from build123d import *

# Parameters (mm, degrees)
BOSS_EXTRUDE1_DEPTH                                 = 6.35
BOSS_EXTRUDE1_DEPTH_BACK                            = 0.762
BOSS_EXTRUDE2_DEPTH                                 = 42.418
CSK_FOR_1_4_FLAT_HEAD_MACHINE_SCREW_100_D           = 6.7564
CSK_FOR_1_4_FLAT_HEAD_MACHINE_SCREW_100_CSINK_D     = 14.3913352
CSK_FOR_1_4_FLAT_HEAD_MACHINE_SCREW_100_CSINK_ANGLE = 100
FILLET1_R                                           = 1.27
CHAMFER1_SIZE                                       = 1.27
FILLET2_R                                           = 1.27


with BuildPart() as part:
    # Sketch2 → Boss-Extrude1 (new, two sides: drawn at the far end of the back side and taken through both)
    with BuildSketch(Plane(origin=(0, 43.18, 0), x_dir=(1, 0, 0), z_dir=(0, 1, 0)).offset(-BOSS_EXTRUDE1_DEPTH_BACK)):
        with BuildLine():
            Line((-27.94, 15.875), (-27.94, -15.875))
            ThreePointArc((-27.94, -15.875), (-24.406243315, -24.406243315), (-15.875, -27.94))
            Line((-15.875, -27.94), (15.875, -27.94))
            ThreePointArc((15.875, -27.94), (24.406243315, -24.406243315), (27.94, -15.875))
            Line((27.94, -15.875), (27.94, 15.875))
            ThreePointArc((27.94, 15.875), (24.406243315, 24.406243315), (15.875, 27.94))
            Line((15.875, 27.94), (-15.875, 27.94))
            ThreePointArc((-15.875, 27.94), (-24.406243315, 24.406243315), (-27.94, 15.875))
        make_face()
    extrude(amount=BOSS_EXTRUDE1_DEPTH + BOSS_EXTRUDE1_DEPTH_BACK)

    # Sketch1 → Boss-Extrude2 (add)
    with BuildSketch(Plane(origin=(0, 0, 0), x_dir=(1, 0, 0), z_dir=(0, 1, 0))):
        with BuildLine():
            Line((-27.94, -15.875), (-27.94, 15.875))
            ThreePointArc((-27.94, 15.875), (-24.406243315, 24.406243315), (-15.875, 27.94))
            Line((-15.875, 27.94), (15.875, 27.94))
            ThreePointArc((15.875, 27.94), (24.406243315, 24.406243315), (27.94, 15.875))
            Line((27.94, 15.875), (27.94, -15.875))
            ThreePointArc((27.94, -15.875), (24.406243315, -24.406243315), (15.875, -27.94))
            Line((15.875, -27.94), (-15.875, -27.94))
            ThreePointArc((-15.875, -27.94), (-24.406243315, -24.406243315), (-27.94, -15.875))
        make_face()
        with BuildLine():
            Line((-22.86, -15.875), (-22.86, 15.875))
            ThreePointArc((-22.86, 15.875), (-20.814140867, 20.814140867), (-15.875, 22.86))
            Line((-15.875, 22.86), (15.875, 22.86))
            ThreePointArc((15.875, 22.86), (20.814140867, 20.814140867), (22.86, 15.875))
            Line((22.86, 15.875), (22.86, -15.875))
            ThreePointArc((22.86, -15.875), (20.814140867, -20.814140867), (15.875, -22.86))
            Line((15.875, -22.86), (-15.875, -22.86))
            ThreePointArc((-15.875, -22.86), (-20.814140867, -20.814140867), (-22.86, -15.875))
        make_face(mode=Mode.SUBTRACT)
    extrude(amount=BOSS_EXTRUDE2_DEPTH)

    # CSK for 1/4 Flat Head Machine Screw (100)1 (through all)
    with Locations(Plane(origin=(0, 49.53, 0), x_dir=(1, 0, 0), z_dir=(0, 1, 0))):
        with Locations((0, 0)):
            CounterSinkHole(CSK_FOR_1_4_FLAT_HEAD_MACHINE_SCREW_100_D / 2, CSK_FOR_1_4_FLAT_HEAD_MACHINE_SCREW_100_CSINK_D / 2, counter_sink_angle=CSK_FOR_1_4_FLAT_HEAD_MACHINE_SCREW_100_CSINK_ANGLE)

    # Fillet1
    fillet1_edges = [part.edges().sort_by_distance(p)[0] for p in [
        (24.406243315, 49.53, 24.406243315),
        (27.94, 49.53, 0),
        (24.406243315, 49.53, -24.406243315),
        (0, 49.53, -27.94),
        (-24.406243315, 49.53, -24.406243315),
        (-27.94, 49.53, 0),
        (-24.406243315, 49.53, 24.406243315),
        (0, 49.53, 27.94),
    ]]
    fillet(fillet1_edges, radius=FILLET1_R)

    # Chamfer1
    chamfer1_edges = [part.edges().sort_by_distance(p)[0] for p in [
        (-22.86, 0, 0),
        (-20.814140867, 0, 20.814140867),
        (0, 0, 22.86),
        (20.814140867, 0, 20.814140867),
        (22.86, 0, 0),
        (20.814140867, 0, -20.814140867),
        (0, 0, -22.86),
        (-20.814140867, 0, -20.814140867),
    ]]
    chamfer(chamfer1_edges, length=CHAMFER1_SIZE)

    # Fillet2
    fillet2_edges = [part.edges().sort_by_distance(p)[0] for p in [
        (-27.94, 0, 0),
        (-24.406243315, 0, -24.406243315),
        (0, 0, -27.94),
        (24.406243315, 0, -24.406243315),
        (27.94, 0, 0),
        (24.406243315, 0, 24.406243315),
        (0, 0, 27.94),
        (-24.406243315, 0, 24.406243315),
    ]]
    fillet(fillet2_edges, radius=FILLET2_R)


solid = part.part
Check sheet for the modelled part. Datum: model origin and axes. Units: mm. A direction names the side the tool comes from. Round coordinates to 2 decimals unless told otherwise and drop trailing zeros. Write each loop counter-clockwise with the first axis right and the second up, starting at its lowest first coordinate (ties: lowest second). Pieces come first, ordered by that corner, then holes. Notation, with made-up numbers: (75, -11.5) -> (121, -11.5) arc R22 cw to (121, 18.5) -> close; hole circle Ø3 at (-33.5, 39). An arc over 180 degrees is marked (long way). Answer as CSV lines item,"result". Start each with the question number.
1) Go/stop test with flat-tipped pins: P1, Ø6, axis at x = 3, z = -2, coming from the +Y side; P2, Ø1, axis at x = 2.5, z = 14, coming from the -Y side. Record where each tip stops, or that it passes through.
2) Section check A-A on x = 0. Enter the section's corners in (y, z), and give its area (3 significant figures).
3) Section check D-D on x = 8. Enter the section's corners in (y, z), and give its area (3 significant figures).
4) Tool access check on faces 1 (the conical face through (-21.01, 1.07, -20.9)), 2 (the conical face through (-3.3, 46.5, 1.4)). Record the directions out of +Z, -Z, +X, -X, +Y, -Y that give a thin tool (end or side, any length) a straight path to the whole face; none if there is none.
5) Section check C-C on y = 23.5. Enter the section's corners in (x, z) (3 decimals).
6) Material ranges on line 1 (Z direction, x = 10, y = 18.5); line 2 (Z direction, x = 0, y = 43), recorded low to high. Write a range as from..to.
7) Section check B-B on z = 0. Enter the section's corners in (x, y).
8) Release check for a two-part mould opening along X. For faces 3 (the flat face through (26, 0, 0)), 4 (the cylindrical face through (24.31, 24.44, -24.5)), 5 (the flat face through (0, 22, -22.86)) record: pulls with the +X half, pulls with the -X half, needs draft (parallel to the pull), parting line crosses it, or undercut.
Found:
1,P1,"stops at y = 49.03"
1,P2,"stops at y = 42.42"
2,outline,"(0, -26.67) arc R1.27 ccw to (1.27, -27.94) -> (48.26, -27.94) arc R1.27 ccw to (49.53, -26.67) -> (49.53, -7.2) -> (46.33, -3.38) -> (42.42, -3.38) -> (42.42, -22.86) -> (1.27, -22.86) -> (0, -24.13) -> close; (0, 24.13) -> (1.27, 22.86) -> (42.42, 22.86) -> (42.42, 3.38) -> (46.33, 3.38) -> (49.53, 7.2) -> (49.53, 26.67) arc R1.27 ccw to (48.26, 27.94) -> (1.27, 27.94) arc R1.27 ccw to (0, 26.67) -> close"
2,area,"765 mm^2"
3,outline,"(0, -26.67) arc R1.27 ccw to (1.27, -27.94) -> (48.26, -27.94) arc R1.27 ccw to (49.53, -26.67) -> (49.53, 26.67) arc R1.27 ccw to (48.26, 27.94) -> (1.27, 27.94) arc R1.27 ccw to (0, 26.67) -> (0, 24.13) -> (1.27, 22.86) -> (42.42, 22.86) -> (42.42, -22.86) -> (1.27, -22.86) -> (0, -24.13) -> close"
3,area,"825 mm^2"
4,face 1,"-Y"
4,face 2,"+Y"
5,outline,"(-27.94, -15.875) arc R12.065 ccw to (-15.875, -27.94) -> (15.875, -27.94) arc R12.065 ccw to (27.94, -15.875) -> (27.94, 15.875) arc R12.065 ccw to (15.875, 27.94) -> (-15.875, 27.94) arc R12.065 ccw to (-27.94, 15.875) -> close; hole (-22.86, -15.875) arc R6.985 ccw to (-15.875, -22.86) -> (15.875, -22.86) arc R6.985 ccw to (22.86, -15.875) -> (22.86, 15.875) arc R6.985 ccw to (15.875, 22.86) -> (-15.875, 22.86) arc R6.985 ccw to (-22.86, 15.875) -> close"
6,line 1,"z = -27.94..-22.86, 22.86..27.94"
6,line 2,"z = -27.94..-3.38, 3.38..27.94"
7,outline,"(-27.94, 1.27) arc R1.27 ccw to (-26.67, 0) -> (-24.13, 0) -> (-22.86, 1.27) -> (-22.86, 42.42) -> (-3.38, 42.42) -> (-3.38, 46.33) -> (-7.2, 49.53) -> (-26.67, 49.53) arc R1.27 ccw to (-27.94, 48.26) -> close; (3.38, 42.42) -> (22.86, 42.42) -> (22.86, 1.27) -> (24.13, 0) -> (26.67, 0) arc R1.27 ccw to (27.94, 1.27) -> (27.94, 48.26) arc R1.27 ccw to (26.67, 49.53) -> (7.2, 49.53) -> (3.38, 46.33) -> close"
8,face 3,"needs draft"
8,face 4,"pulls with the +X half"
8,face 5,"undercut"
